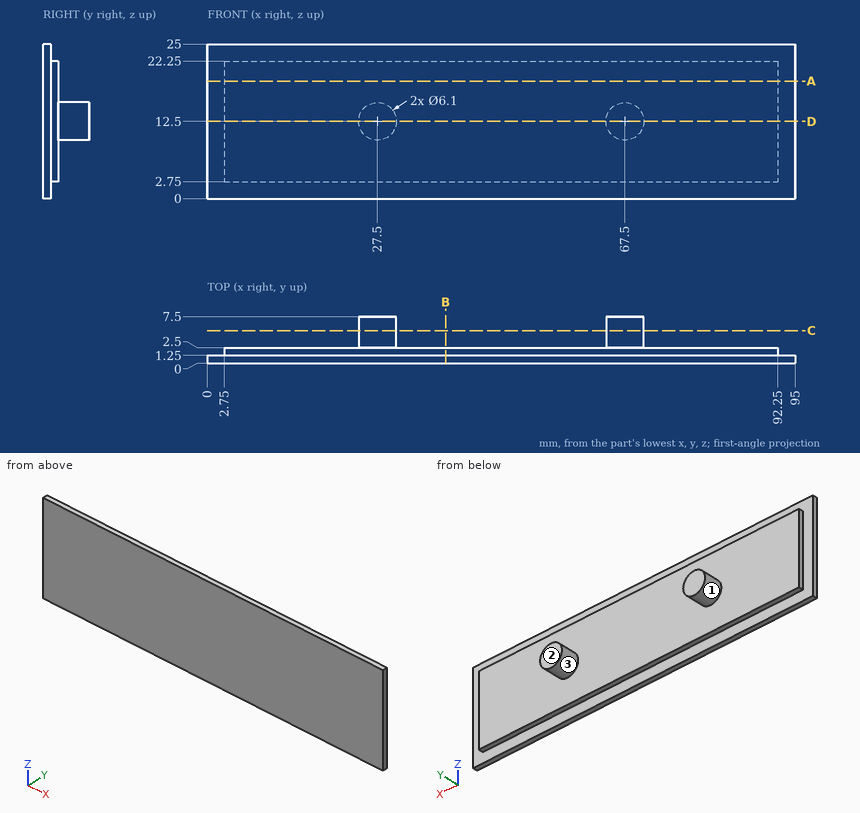
Part print with two shaded views. Sizes in mm from the minimum x, y, z corner. Round coordinates to 2 decimals unless told otherwise and drop trailing zeros. Write each loop counter-clockwise with the first axis right and the second up, starting at its lowest first coordinate (ties: lowest second). Pieces come first, ordered by that corner, then holes. Notation, with made-up numbers: (7, 30) - (14, 30) arc R32 cw to (14, 57) - close; hole circle Ø2 at (46, 36.25). An arc over 180 degrees is marked (long way). Use CSV: the item, a comma, the result in double quotes.
Item 1: Slice it at B-B, the plane x = 38.5. Write the cut outline in (y, z), then the cut area to 3 significant figures.
Results list:
outline,"(0, 0) - (1.25, 0) - (1.25, 2.75) - (2.5, 2.75) - (2.5, 22.25) - (1.25, 22.25) - (1.25, 25) - (0, 25) - close"
area,"55.6 mm²"
Item 2: Slice it at C-C, the plane y = 5.25. Write the cut outline in (x, z), then the cut area to 3 significant figures.
Results list:
outline,"circle Ø6.1 at (27.5, 12.5); circle Ø6.1 at (67.5, 12.5)"
area,"58.4 mm²"
Item 3: Flat gauge pins, fed straight in: P1, Ø1.4, axis at y = 2, z = 12.5, coming from the +X side; P2, Ø2, axis at y = 2.5, z = 15.5, coming from the -X side; P3, Ø6, axis at x = 57.5, z = 9.5, coming from the +Y side. Where does each tip first touch, or does it go through?
Results list:
P1,"stops at x = 92.25"
P2,"stops at x = 2.75"
P3,"stops at y = 2.5"
Item 4: Slice it at A-A, the plane z = 19. Write the cut outline in (x, y).
Results list:
outline,"(0, 0) - (95, 0) - (95, 1.25) - (92.25, 1.25) - (92.25, 2.5) - (2.75, 2.5) - (2.75, 1.25) - (0, 1.25) - close"
Item 5: Pull direction X, two halves, no side cores. Call the marked faces 1, 2 and 3: pulls with the +X half, pulls with the -X half, needs draft (parallel to the pull), parting line crosses it, or undercut.
Results list:
face 1,"undercut"
face 2,"needs draft"
face 3,"undercut"
Item 6: Wall check: L1, parallel to X at y = 1.75, z = 17; L2, parallel to Y at x = 48, z = 21.25; L3, parallel to Y at x = 63.5, z = 22.5. Give the ranges that are in metal, low to high.
Results list:
L1,"x = 2.75 to 92.25"
L2,"y = 0 to 2.5"
L3,"y = 0 to 1.25"
Item 7: Slice it at D-D, the plane z = 12.5. Write the cut outline in (x, y).
Results list:
outline,"(0, 0) - (95, 0) - (95, 1.25) - (92.25, 1.25) - (92.25, 2.5) - (70.55, 2.5) - (70.55, 7.5) - (64.45, 7.5) - (64.45, 2.5) - (30.55, 2.5) - (30.55, 7.5) - (24.45, 7.5) - (24.45, 2.5) - (2.75, 2.5) - (2.75, 1.25) - (0, 1.25) - close"
